Design review of the part built by this model. Coordinates are the model's own, in mm. Face numbers are marked on the shaded views. Round coordinates to 2 decimals unless told otherwise and drop trailing zeros. Loops run counter-clockwise (first coordinate to the right, second up) from the corner with the lowest first, then second, coordinate; pieces in that order, holes last. Notation, with made-up numbers: (75.5, -38.75) - (100.5, -38.75) arc R15 cw to (100.5, -9.75) - close; hole circle Ø5 at (75, 6). An arc over 180 degrees is marked (long way). Return JSON: item names as keys, results as strings. Group by question number.
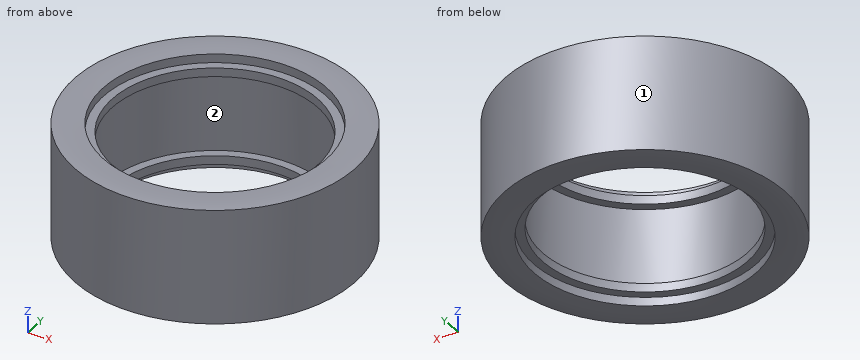
from build123d import *


with BuildPart() as part:
    # Sketch1 → Revolve1 (revolve)
    with BuildSketch(Plane(origin=(0, 0, 0), x_dir=(1, 0, 0), z_dir=(0, 1, 0))):
        with BuildLine():
            Line((25.75, 226.600121105), (25.75, 224.600121105))
            Line((25.75, 224.600121105), (23.75, 224.600121105))
            Line((23.75, 224.600121105), (23.75, 222.600121105))
            Line((23.75, 222.600121105), (25.75, 222.600121105))
            Line((25.75, 222.600121105), (25.75, 204.100121105))
            Line((25.75, 204.100121105), (23.75, 204.100121105))
            Line((23.75, 204.100121105), (23.75, 202.100121105))
            Line((23.75, 202.100121105), (25.75, 202.100121105))
            Line((25.75, 202.100121105), (25.75, 200.100121105))
            add(Edge.make_bspline(
                [(25.75, 200.100121105), (28.665236828, 199.927378107), (31.106495402, 199.927378107), (32.45, 200.100121105)],
                knots=[0, 0, 0, 0, 1, 1, 1, 1], degree=3))
            Line((32.45, 200.100121105), (32.45, 226.600121105))
            add(Edge.make_bspline(
                [(25.75, 226.600121105), (28.665236828, 226.772864103), (31.106495402, 226.772864103), (32.45, 226.600121105)],
                knots=[0, 0, 0, 0, 1, 1, 1, 1], degree=3))
        make_face()
    revolve(axis=Axis((0, 0, 0), (0, 0, -1)))


solid = part.part
Q1. For line 1 (Y direction, x = 0, z = -201.3); line 2 (X direction, y = 0, z = -203.2), list the stretches that pass through material, from the lowest coordinate up.
Q2. Insertion check: pin 1 Ø1.5 at (y, z) = (-17, -214) entering from +X; pin 2 Ø5 at (x, z) = (8.5, -219.5) entering from +Y; pin 3 Ø10 at (y, z) = (-22.5, -211) entering from +X; pin 4 Ø2 at (x, y) = (-4.5, -20.5) entering from -Z. Each pin has a flat end and moves straight along its axis. Give the tip position at first contact, or say it passes through.
Q3. Draft analysis for pull direction X (two halves, no side actions). For the marked faces 1 and 2, state which applies: pulls with the +X half, pulls with the -X half, needs draft (parallel to the pull), parting line crosses it, or undercut.
Q4. Add section A-A, the plane z = -213. State the section outline as (x, y) points.
Evaluation:
{
 "1": {"line 1": "-32.45 to -25.75, 25.75 to 32.45", "line 2": "-32.45 to -23.75, 23.75 to 32.45"},
 "2": {"pin 1": "x = 28.09", "pin 2": "y = 31.89", "pin 3": "x = 27.33", "pin 4": "through"},
 "3": {"face 1": "parting line crosses it", "face 2": "undercut"},
 "4": {"outline": "circle Ø64.9 at (0, 0); hole circle Ø51.5 at (0, 0)"}
}
